Build history of the part. All positions in model axes, mm. Face numbers are marked on the shaded views. A direction names the side the tool comes from. Give positions to 0.01 mm unless a question says otherwise; leave off trailing zeros. Write each loop counter-clockwise with the first axis right and the second up, starting at its lowest first coordinate (ties: lowest second). Pieces come first, ordered by that corner, then holes. Notation, with made-up numbers: (-7.75, 56.25) -> (10.25, 56.25) arc R20 ccw to (10.25, 88.25) -> close; hole circle Ø10 at (79.5, -16.5). An arc over 180 degrees is marked (long way). One line per question, with ' | ' between items. Start each with the question number.
(1) Band-saw the part on B-B, the plane y = 5.5. Give the cut face in (x, z).
(2) Drill centre lines: probe 1 along Z at (x, y) = (-6, 5.75); probe 2 along X at (y, z) = (2, 3.75); probe 3 along X at (y, z) = (8.25, -2.5). Where is each one in solid material? Low to high. Write a range as from..to.
(3) Pin check, flat tips, straight feed: P1, Ø1.6, axis at y = 6, z = 1.5, coming from the -X side; P2, Ø1, axis at x = 5, z = -0.5, coming from the +Y side; P3, Ø0.5, axis at x = -5, z = -4, coming from the +Y side; P4, Ø2, axis at y = 6.5, z = 1.5, coming from the +X side. Stop position of each tip, or through.
(4) Band-saw the part on C-C, the plane z = -2.5. Give the cut face in (x, y).
(5) Band-saw the part on D-D, the plane x = -0.5. Give the cut face in (y, z), and give its area (3 significant figures).
(6) Tool access for the marked faces 5, 6 and 7: list every direction of +Z, -Z, +X, -X, +Y, -Y with a clear straight run to the whole face (end or side of a thin tool).
(7) Pull direction X, two halves, no side cores. Call the marked faces 1, 2, 3 and 4: released by +X, released by -X, zero draft, split by the parting line, or undercut.
(8) Band-saw the part on A-A, the plane y = 7.5. Give the cut face in (x, z), and give its area (4 significant figures).
from build123d import *

# Parameters (mm, degrees)
BOSS_EXTRUDE1_DEPTH = 9
SKETCH2_W           = 2
SKETCH2_H           = 2
CUT_EXTRUDE1_DEPTH  = 9
CUT_EXTRUDE2_DEPTH  = 8
CUT_EXTRUDE3_DEPTH  = 8
CUT_EXTRUDE4_DEPTH  = 8
CUT_EXTRUDE5_DEPTH  = 8


with BuildPart() as part:
    # Sketch1 → Boss-Extrude1 (new body)
    with BuildSketch(Plane(origin=(0, 0, 0), x_dir=(1, 0, 0), z_dir=(0, 1, 0))):
        Polygon((-8, 4.5), (-8, 0.5), (-6, -1.5), (-2, -2.5), (-2, -4.5), (8, -4.5), (8, 4.5), align=None)
    extrude(amount=BOSS_EXTRUDE1_DEPTH)

    # Sketch2 → Cut-Extrude1 (cut)
    with BuildSketch(Plane.XY.offset(4.5)):
        with Locations((5, 8)):
            Rectangle(SKETCH2_W, SKETCH2_H)
        Polygon((-8, 6), (-4, 6), (-2, 8), (0, 9), (-8, 9), align=None)
        Polygon((-8, 2), (-6, 0), (-8, 0), align=None)
    extrude(amount=-CUT_EXTRUDE1_DEPTH, mode=Mode.SUBTRACT)

    # Sketch4 → Cut-Extrude2 (cut)
    with BuildSketch(Plane.XY.offset(4.5)):
        Polygon((-4, 6), (-8, 2), (-8, 6), align=None)
    extrude(amount=-CUT_EXTRUDE2_DEPTH, mode=Mode.SUBTRACT)

    # 3DSketch1 → Cut-Extrude3 (cut, along a direction that is not the sketch's normal)
    with BuildSketch(Plane(origin=(8, 0, 4.5), x_dir=(-0.5121475197315839, 0.7682212795973759, -0.3841106397986879), z_dir=(0, -0.447213595499958, -0.894427190999916))):
        Polygon((0, 0), (1.024295039, -1.717795003), (6.913991516, -2.862991672), (11.715374514, 0), (8.642489395, 5.153385009), align=None)
    extrude(amount=-CUT_EXTRUDE3_DEPTH, dir=(0, 0, -1), mode=Mode.SUBTRACT)

    # 3DSketch2 → Cut-Extrude4 (cut, along a direction that is not the sketch's normal)
    with BuildSketch(Plane(origin=(-2, 0, 4.5), x_dir=(0.5773502691896258, 0.5773502691896258, -0.5773502691896257), z_dir=(0.7071067811865476, -0.7071067811865476, 0))):
        Polygon((0, 0), (4.618802154, 3.265986324), (6.92820323, 0), (1.154700538, -1.632993162), align=None)
    extrude(amount=-CUT_EXTRUDE4_DEPTH, dir=(0, -1, 0), mode=Mode.SUBTRACT)

    # 3DSketch3 → Cut-Extrude5 (cut, along a direction that is not the sketch's normal)
    with BuildSketch(Plane(origin=(-2, 8, -3.5), x_dir=(-0.3903600291794133, -0.7807200583588266, 0.48795003647426655), z_dir=(-0.19611613513818413, 0.5883484054145521, 0.7844645405527362))):
        Polygon((0, 0), (8.490330635, -2.985680109), (10.246950766, 0), (9.173460686, 3.980906812), (3.513240263, 5.971360218), align=None)
    extrude(amount=CUT_EXTRUDE5_DEPTH, dir=(0, 1, 0), mode=Mode.SUBTRACT)


solid = part.part
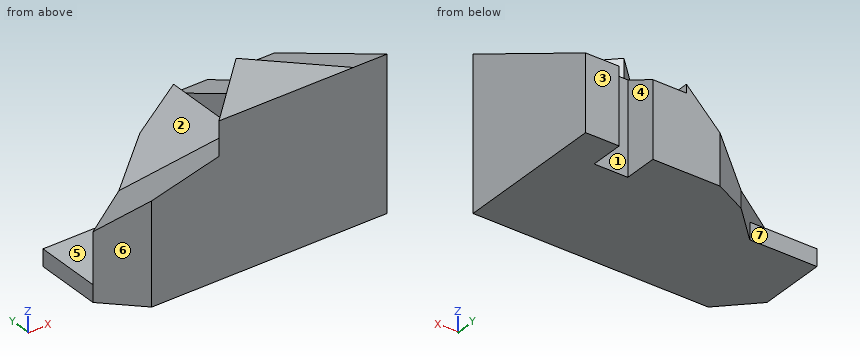
Results:
1) outline: (-8, -4.5) -> (8, -4.5) -> (8, 1.75) -> (2, 1.75) -> (2, 0.5) -> (0.5, -1) -> (-4.5, -2.25) -> (-4.5, -3.5) -> (-8, -3.5) -> close
2) probe 1: z = -4.5..-3.5 | probe 2: x = 0..4 | probe 3: x = -1..4, 6..8
3) P1: stops at x = 2 | P2: stops at y = 7 | P3: stops at y = 6 | P4: stops at x = 8
4) outline: (-8, 2) -> (-6, 0) -> (8, 0) -> (8, 9) -> (6, 9) -> (6, 7) -> (4, 7) -> (4, 9) -> (0, 9) -> (-1, 8.5) -> (-1, 7) -> (-4, 6) -> close
5) outline: (0, -4.5) -> (8.75, -4.5) -> (8.75, -2) -> (6.5, -2) -> (1.5, 1.75) -> (1.5, 4.5) -> (0, 4.5) -> close | area: 41.0 mm²
6) face 5: +Z, -X, +Y | face 6: +Z, -Z, -X, -Y | face 7: +Z, -Z, -X, +Y
7) face 1: undercut | face 2: released by -X | face 3: zero draft | face 4: undercut
8) outline: (-2.5, -4.5) -> (4, -4.5) -> (4, 0.75) -> (2, 0.75) -> (2, 0.5) -> (-1.5, -3) -> (-2.5, -3.25) -> close; (6, -4.5) -> (8, -4.5) -> (8, 0.75) -> (6, 0.75) -> close | area: 33.75 mm²
